The listing builds one solid part. Answer for the finished solid, in the listing's coordinates (mm). Round coordinates to 2 decimals unless told otherwise and drop trailing zeros. Order: outer loops, then holes, each group sorted by start corner. A loop starts at its lowest first (then second) coordinate and runs counter-clockwise, first axis right, second up. Notation, with made-up numbers: M 8,73 L 21,73 A24 cw 21,103 Z; hole C 16,6.5 d10. An arc over 180 degrees is marked long. Write item = value, one per line. Start each with the question number.
(1) A cutting plane is placed at A-A, the plane x = 0. Determine the outline of the cut face in (y, z), and give its area (3 significant figures).
(2) This flat-tipped pin is pushed along its axis until it touches: pin 1 (1 mm diameter, centred on x = 2.5, z = 1, fed in from +Y). Where does it stop, or does it pass through?
(3) For a pull along Y with two mould halves and no side action, classify faces 1 (the face through (1.66, -12.8, -0.07)), 2 (the face through (-0.088, 17.167, -0.07)), 3 (the face through (-4, 0, 0)) as released by +Y, released by -Y, zero draft, split by the parting line, or undercut.
(4) A cutting plane is placed at B-B, the plane z = 1.5. Determine the outline of the cut face in (x, y), and give its area (3 significant figures).
(5) Straight lines are drawn through the part: probe 1 along Y at (x, z) = (0, 0); probe 2 along Y at (x, z) = (-1, -0.25); probe 3 along X at (y, z) = (12.5, -3.5). For each, find the intervals that lie inside material, in ascending order. Write a range as from..to.
(6) A cutting plane is placed at C-C, the plane x = -2.75. Determine the outline of the cut face in (y, z).
Autodesk Inventor part; units mm, degrees
ref_plane "YZ Plane" through (0, 0, 0) normal (1, 0, 0) x (0, 1, 0)
ref_plane "XZ Plane" through (0, 0, 0) normal (0, 1, 0) x (-1, 0, 0)
ref_plane "XY Plane" through (0, 0, 0) normal (0, 0, 1) x (1, 0, 0)
sketch "Sketch1" plane through (0, 0, 0) normal (0, 0, 1) x (1, 0, 0)
  line L0 (0, 17.1679) -> (0, 17.1679)
  line L1 (4, 13.1679) -> (4, -13.1679)
  line L2 (0, -17.1679) -> (0, -17.1679)
  line L3 (-4, -13.1679) -> (-4, 13.1679)
  line L4 (-4, 17.1679) -> (0, 17.1679) construction
  line L5 (0, 17.1679) -> (0, 0) construction
  line L6 (0, 0) -> (-4, 0) construction
  line L7 (-4, 0) -> (-4, 17.1679) construction
  arc A0 (4, 13.1679) -> (0, 17.1679) centre (0, 13.1679) ccw
  arc A1 (0, 17.1679) -> (-4, 13.1679) centre (0, 13.1679) ccw
  arc A2 (-4, -13.1679) -> (0, -17.1679) centre (0, -13.1679) ccw
  arc A3 (0, -17.1679) -> (4, -13.1679) centre (0, -13.1679) ccw
  dimension "d0" = 4
  dimension "d6" = 26.3358
extrude "Extrusion1" add sketch "Sketch1" along normal mid plane 10
sketch "Sketch2" plane through (0, 0, 5) normal (0, 0, 1) x (1, 0, 0)
  arc A0 (4, 13.1679) -> (-4, 13.1679) centre (0, 13.1679) ccw construction
  arc A1 (-4, -13.1679) -> (4, -13.1679) centre (0, -13.1679) ccw construction
  point P0 (0, 0)
hole "Hole1" at (0, 13.1679, 5) at (0, -13.1679, 5) direction (0, 0, -1) diameter 3.4 end through all
equation "\"d6\" = LengthF"
properties part number "F"
Reported:
q1.outline = M -17.17,-5 L -14.87,-5 L -14.87,5 L -17.17,5 Z; M -11.47,-5 L 11.47,-5 L 11.47,5 L -11.47,5 Z; M 14.87,-5 L 17.17,-5 L 17.17,5 L 14.87,5 Z
q1.area = 275 mm²
q2.pin_1 = 16.63
q3.face_1 = undercut
q3.face_2 = released by +Y
q3.face_3 = zero draft
q4.outline = M -4,-13.17 A4 ccw 4,-13.17 L 4,13.17 A4 ccw -4,13.17 Z; hole C 0,-13.17 d3.4; hole C 0,13.17 d3.4
q4.area = 243 mm²
q5.probe_1 = -17.17..-14.87, -11.47..11.47, 14.87..17.17
q5.probe_2 = -17.04..-14.54, -11.79..11.79, 14.54..17.04
q5.probe_3 = -4..-1.56, 1.56..4
q6.outline = M -16.07,-5 L 16.07,-5 L 16.07,5 L -16.07,5 Z
